```python
from build123d import *

# Parameters (mm, degrees)
F1_DEPTH = 6
F0_R     = 9.5
F2_DEPTH = 8


with BuildPart() as f1:
    # F0 (on Front) → F1 (new body, symmetric)
    with BuildSketch(Plane.XZ):
        with BuildLine():
            ThreePointArc((8.394908, -14.782609), (0, -17), (-8.394908, -14.782609))
            ThreePointArc((-8.394908, -14.782609), (-5.556767, -21.532262), (-11.357817, -26))
            Line((-11.357817, -26), (-17, -26))
            Line((-17, -26), (-17, -36))
            Line((-17, -36), (-12, -36))
            Line((-12, -36), (-12, -31))
            Line((-12, -31), (12, -31))
            Line((12, -31), (12, -36))
            Line((12, -36), (17, -36))
            Line((17, -36), (17, -26))
            Line((17, -26), (11.357817, -26))
            ThreePointArc((11.357817, -26), (5.556767, -21.532262), (8.394908, -14.782609))
        make_face()
    extrude(amount=F1_DEPTH, both=True)

    # F0 (on Front) → F2 (join, symmetric)
    with BuildSketch(Plane.XZ):
        with BuildLine():
            ThreePointArc((8.394908, -14.782609), (14.692063, -8.552385), (17, 0))
            ThreePointArc((17, 0), (-8.552385, 14.692063), (-8.394908, -14.782609))
            ThreePointArc((-8.394908, -14.782609), (0, -17), (8.394908, -14.782609))
        make_face()
        Circle(F0_R, mode=Mode.SUBTRACT)
    extrude(amount=F2_DEPTH, both=True)


solid = f1.part
```
Work out the finished part from the listing and answer in its coordinate system (mm). A direction names the side the tool comes from. Round coordinates to 2 decimals unless told otherwise and drop trailing zeros. Loops run counter-clockwise (first coordinate to the right, second up) from the corner with the lowest first, then second, coordinate; pieces in that order, holes last.
(1) Find the intervals of material crossed by L1, parallel to Z at x = -6, y = -4.5; L2, parallel to Z at x = 0, y = 4.5; L3, parallel to Z at x = -6.5, y = 4, in increasing order.
Computed values:
L1: z = -31 to -22.7, -17.3 to -7.37, 7.37 to 15.91
L2: z = -31 to -9.5, 9.5 to 17
L3: z = -31 to -23.52, -16.48 to -6.93, 6.93 to 15.71
(2) For faces 1 (the flat face through (12, 0, -33)), 2 (the flat face through (-14, 0, -26)), 3 (the flat face through (14, 0, -26)), determine the directions among +Z, -Z, +X, -X, +Y, -Y from which every point of the face is accessible in a straight line to the end or side of a thin tool.
Computed values:
face 1: -Z, +Y, -Y
face 2: -X, +Y, -Y
face 3: +X, +Y, -Y
(3) The part is cut by section D-D, the plane z = -13. Give the vertices of the cut face in (x, y).
Computed values:
outline: (-10.95, -8) - (10.95, -8) - (10.95, 8) - (-10.95, 8) - close
(4) The part is cut by section A-A, the plane x = 0. Give the vertices of the cut face in (y, z).
Computed values:
outline: (-8, -17) - (-6, -17) - (-6, -31) - (6, -31) - (6, -17) - (8, -17) - (8, -9.5) - (-8, -9.5) - close; (-8, 9.5) - (8, 9.5) - (8, 17) - (-8, 17) - close
(5) The part is cut by section C-C, the plane x = -6. Give the vertices of the cut face in (y, z).
Computed values:
outline: (-8, -15.91) - (-6, -15.91) - (-6, -17.3) - (6, -17.3) - (6, -15.91) - (8, -15.91) - (8, -7.37) - (-8, -7.37) - close; (-8, 7.37) - (8, 7.37) - (8, 15.91) - (-8, 15.91) - close; (-6, -31) - (6, -31) - (6, -22.7) - (-6, -22.7) - close
(6) The mould has two halves that part along Z. Classify faces 4 (the flat face through (-15, 0, -36)), 5 (the cylindrical face through (5.586, -0.084, -21.639)), 6 (the flat face through (-12, 0, -34)), 7 (the cylindrical face through (4.38, 0.11, -8.43)): pulls with the +Z half, pulls with the -Z half, needs draft (parallel to the pull), parting line crosses it, or undercut.
Computed values:
face 4: pulls with the -Z half
face 5: undercut
face 6: needs draft
face 7: undercut
(7) The part is cut by section B-B, the plane y = -1. Give the vertices of the cut face in (x, z).
Computed values:
outline: (-17, -36) - (-12, -36) - (-12, -31) - (12, -31) - (12, -36) - (17, -36) - (17, -26) - (11.36, -26) arc R6 cw to (8.39, -14.78) arc R17 ccw (long way) to (-8.39, -14.78) arc R6 cw to (-11.36, -26) - (-17, -26) - close; hole circle Ø19 at (0, 0)
(8) Each of these flat-tipped pins is pushed along its axis until it touches: P1, Ø17, axis at x = -6, z = -20, coming from the -Y side; P2, Ø6, axis at y = -2, z = -17.5, coming from the +X side; P3, Ø5, axis at x = -8.5, y = 2, coming from the -Z side; P4, Ø6, axis at y = -4.5, z = -15.5, coming from the +X side. Where does it stop, or does it pass through?
Computed values:
P1: stops at y = -8
P2: stops at x = 8.87
P3: stops at z = -31
P4: stops at x = 11.52
